For this review, take the finished solid that the model builds, in its own axes (mm). Face numbers are marked on the shaded views. A direction names the side the tool comes from. Coordinates: 2 decimals unless noted, no trailing zeros. Loops run counter-clockwise (first coordinate to the right, second up) from the corner with the lowest first, then second, coordinate; pieces in that order, holes last. Notation, with made-up numbers: M 15,38 L 40,38 A20 ccw 40,55 Z; hole C 2,-30 d8. An arc over 180 degrees is marked long. Put each result on its own line as item: value.
```python
from build123d import *

# Parameters (mm, degrees)
SKETCH1_W           = 51.5
SKETCH1_H           = 17.6
BOSS_EXTRUDE1_DEPTH = 8.8
SKETCH2_W           = 51.5
SKETCH2_H           = 13.7
CUT_EXTRUDE1_DEPTH  = 5.8
SKETCH3_R           = 1.6
CUT_EXTRUDE2_DEPTH  = 17.8
CHAMFER1_SIZE       = 1
SKETCH4_R           = 3
BOSS_EXTRUDE2_DEPTH = 53
FILLET1_R           = 4


with BuildPart() as part:
    # Sketch1 → Boss-Extrude1 (new body)
    with BuildSketch(Plane.XY):
        with Locations((25.75, 8.8)):
            Rectangle(SKETCH1_W, SKETCH1_H)
    extrude(amount=BOSS_EXTRUDE1_DEPTH)

    # Sketch2 → Cut-Extrude1 (cut)
    with BuildSketch(Plane(origin=(0, 0, 0), x_dir=(-1, 0, 0), z_dir=(0, 0, -1))):
        with Locations((-25.75, 8.8)):
            Rectangle(SKETCH2_W, SKETCH2_H)
    extrude(amount=-CUT_EXTRUDE1_DEPTH, mode=Mode.SUBTRACT)

    # Sketch3 → Cut-Extrude2 (cut)
    with BuildSketch(Plane(origin=(0, 17.6, 0), x_dir=(1, 0, 0), z_dir=(0, 1, 0))):
        with Locations(Location((2.9, -2.9, 0), (0, 0, 270))):
            Circle(SKETCH3_R)
        with Locations(Location((48.6, -2.9, 0), (0, 0, 270))):
            Circle(SKETCH3_R)
    extrude(amount=-CUT_EXTRUDE2_DEPTH, mode=Mode.SUBTRACT)

    # Chamfer1
    chamfer1_edges = [part.edges().sort_by_distance(p)[0] for p in [
        (2.9, 17.6, 1.3),
        (48.6, 17.6, 1.3),
    ]]
    chamfer(chamfer1_edges, length=CHAMFER1_SIZE)

    # Sketch4 → Boss-Extrude2 (add)
    with BuildSketch(Plane.XY.offset(8.8)):
        with Locations(Location((25.75, 8.8, 0), (0, 0, 180))):
            Circle(SKETCH4_R)
    extrude(amount=BOSS_EXTRUDE2_DEPTH)

    # Fillet1
    fillet1_edges = [part.edges().sort_by_distance(p)[0] for p in [
        (28.75, 8.8, 8.8),
    ]]
    fillet(fillet1_edges, radius=FILLET1_R)


solid = part.part
```
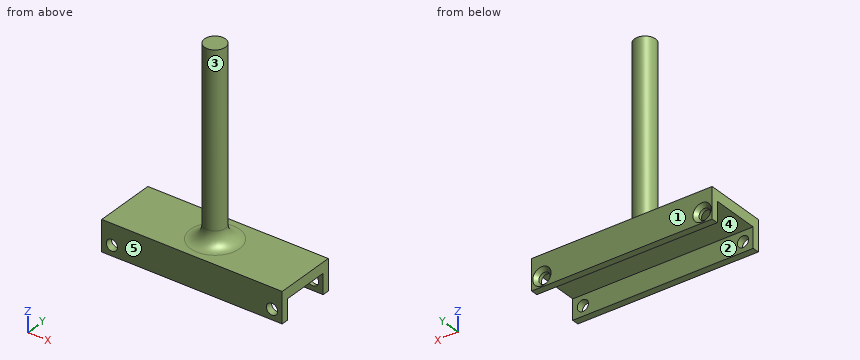
(1) Add section D-D (y = 8.8). Write out the cut boundary in (x, z).
Determined:
outline: M 0,5.8 L 51.5,5.8 L 51.5,8.8 L 32.75,8.8 A4 cw 28.75,12.8 L 28.75,61.8 L 22.75,61.8 L 22.75,12.8 A4 cw 18.75,8.8 L 0,8.8 Z
(2) Wall thickness on line 1 along X through (y, z) = (1.2, 2.9); line 2 along Y through (x, z) = (8, 5); line 3 along Z through (x, y) = (14, 13.5): over which ranges is each line inside the solid? List them lowest first. Write a range as [from, to].
Determined:
line 1: x = [0, 1.3], [4.5, 47], [50.2, 51.5]
line 2: y = [0, 1.95], [15.65, 17.6]
line 3: z = [5.8, 8.8]
(3) For pin 1 (10 mm diameter, centred on y = 4, z = 26, fed in from -X); pin 2 (4 mm diameter, centred on y = 11.5, z = 38.5, fed in from +X); pin 3 (1.5 mm diameter, centred on y = 13.5, z = 26, fed in from -X); pin 4 (4 mm diameter, centred on x = 37.5, y = 7, fed in from +Z), all flat-tipped, find the tip position at first contact; note any pin that passes through.
Determined:
pin 1: stops at x = 22.75
pin 2: stops at x = 28.67
pin 3: passes through
pin 4: stops at z = 8.8
(4) Draft analysis for pull direction Y (two halves, no side actions). For the marked faces 3, 4 and 5, state which applies: +Y half, -Y half, draft (parallel to the pull), parting line (faces both ways), or undercut.
Determined:
face 3: parting line
face 4: undercut
face 5: -Y half
(5) Add section B-B (z = 2.9). Write out the cut boundary in (x, y).
Determined:
outline: M 0,0 L 1.3,0 L 1.3,1.95 L 0,1.95 Z; M 0,15.65 L 1.3,15.65 L 1.3,16.6 L 0.3,17.6 L 0,17.6 Z; M 4.5,0 L 47,0 L 47,1.95 L 4.5,1.95 Z; M 4.5,15.65 L 47,15.65 L 47,16.6 L 46,17.6 L 5.5,17.6 L 4.5,16.6 Z; M 50.2,0 L 51.5,0 L 51.5,1.95 L 50.2,1.95 Z; M 50.2,15.65 L 51.5,15.65 L 51.5,17.6 L 51.2,17.6 L 50.2,16.6 Z
(6) Add section A-A (x = 2.9). Write out the cut boundary in (y, z).
Determined:
outline: M 0,0 L 1.95,0 L 1.95,1.3 L 0,1.3 Z; M 0,4.5 L 1.95,4.5 L 1.95,5.8 L 15.65,5.8 L 15.65,4.5 L 16.6,4.5 L 17.6,5.5 L 17.6,8.8 L 0,8.8 Z; M 15.65,0 L 17.6,0 L 17.6,0.3 L 16.6,1.3 L 15.65,1.3 Z
(7) Tool access review of the marked faces 1 and 2: name each direction out of +Z, -Z, +X, -X, +Y, -Y from which nothing blocks a thin tool from reaching the whole face with its end or side.
Determined:
face 1: +Z, -Z, +X, -X, +Y
face 2: -Z, +X, -X
(8) Add section C-C (x = 25.75). Write out the cut boundary in (y, z), plus the area to 3 significant figures.
Determined:
outline: M 0,0 L 1.95,0 L 1.95,5.8 L 15.65,5.8 L 15.65,0 L 17.6,0 L 17.6,8.8 L 15.8,8.8 A4 cw 11.8,12.8 L 11.8,61.8 L 5.8,61.8 L 5.8,12.8 A4 cw 1.8,8.8 L 0,8.8 Z
area: 400 mm^2
